Model file for the job. Use its own axes, mm. Coordinates: 2 decimals unless noted, no trailing zeros. Order: outer loops, then holes, each group sorted by start corner. A loop starts at its lowest first (then second) coordinate and runs counter-clockwise, first axis right, second up. Notation, with made-up numbers: (23.25, -39.75) -> (36.25, -39.75) arc R12 ccw to (36.25, -26.75) -> close; hole circle Ø6 at (55.5, 88). An arc over 180 degrees is marked (long way). Use CSV: the item, a comma, the result in double quotes. Start each with the question number.
(1) Cut at C-C on y = 97.5. Write the cut outline in (x, z), plus the area to 3 significant figures.
(2) Cut at B-B on x = 26. Write the cut outline in (y, z), plus the area to 3 significant figures.
(3) Pin check, flat tips, straight feed: pin 1 Ø1.5 at (x, y) = (-29.5, 83) entering from -Z; pin 2 Ø1.5 at (y, z) = (94, 2) entering from +X. Stop position of each tip, or through.
(4) Cut at A-A on z = 1.7. Write the cut outline in (x, y), plus the area to 3 significant figures.
(5) Probe L1, parallel to Y at x = -1, z = 0.4; L2, parallel to Y at x = -0.17, z = 1.5; L3, parallel to Y at x = -48, z = 1.15. List the from-to ranges inside material, lowest first.
(6) Pull direction X, two halves, no side cores. Call faces 1 (the flat face through (-85, 53, 1)), 2 (the flat face through (-1, 66, 3)), 3 (the cylindrical face through (-0.645, 115.504, 1.479)): pulls with the +X half, pulls with the -X half, needs draft (parallel to the pull), parting line crosses it, or undercut.
Autodesk Inventor part; units mm, degrees
ref_plane "YZ Plane" through (0, 0, 0) normal (1, 0, 0) x (0, 1, 0)
ref_plane "XZ Plane" through (0, 0, 0) normal (0, 1, 0) x (-1, 0, 0)
ref_plane "XY Plane" through (0, 0, 0) normal (0, 0, 1) x (1, 0, 0)
sketch "Boceto1" plane through (0, 0, 0) normal (0, 0, 1) x (1, 0, 0)
  arc A0 (-1.5, 113.1763) -> (1.5, 113.1763) centre (0, 113.1763) ccw
  line L0 (0, 113.1763) -> (0, 116.1763)
  line L1 (-75, 45) -> (75, 45)
  line L2 (75, 45) -> (85, 45)
  line L3 (-75, 45) -> (-85, 45)
  line L4 (0, 117.735) -> (-0.0114, 117.7429)
  line L5 (-85, 55) -> (0, 111.6763)
  line L6 (0, 111.6763) -> (85, 55)
  line L7 (-2.22, 113.8018) -> (0.2156, 115.4258)
  line L8 (1.8799, 112.9298) -> (0.2156, 115.4258)
  line L9 (-0.5557, 111.3058) -> (1.8799, 112.9298)
  line L10 (1.8799, 112.9298) -> (0.2156, 115.4258)
  line L11 (-2.22, 113.8018) -> (0.2156, 115.4258)
  line L12 (-0.5557, 111.3058) -> (-2.22, 113.8018)
  line L13 (-2.22, 113.8018) -> (1.8799, 112.9298)
  line L14 (-0.5557, 111.3058) -> (0.2156, 115.4258)
  circle A1 centre (-0.17, 113.3658) radius 2.0958
  line L15 (85, 45) -> (85, 59.843)
  line L16 (-85, 45) -> (-85, 59.843)
  circle A2 centre (-0.17, 113.3658) radius 2.1904
  line L17 (0, 117.0317) -> (-85, 60.3554)
  line L18 (85, 60.3554) -> (0, 117.0317)
  line L19 (-85, 60.3554) -> (-85, 45)
  line L20 (85, 45) -> (85, 60.3554)
  point P0 (0, 0)
  point P1 (96.4858, 46.8907)
  point P2 (-94.6783, 48.1668)
  point P3 (-94.6783, 45)
  point P4 (96.4858, 45)
  dimension "d0" = 3
extrude "Extrusión1" add sketch "Boceto1" along normal blind 3 contours A2 L6 L15 L2 L1 L3 L16 L5 | L5 L16 L19 L17 L18 L20 L15 L6 A2
Outcome:
1,outline,"(-29.29, 0) -> (29.29, 0) -> (29.29, 3) -> (-29.29, 3) -> close"
1,area,"176 mm2"
2,outline,"(45, 0) -> (99.7, 0) -> (99.7, 3) -> (45, 3) -> close"
2,area,"164 mm2"
3,pin 1,"z = 0"
3,pin 2,"x = 35.67"
4,outline,"(-85, 45) -> (85, 45) -> (85, 60.36) -> (0, 117.03) -> (-85, 60.36) -> close; hole circle Ø4.38 at (-0.17, 113.37)"
4,area,"7,410 mm2"
5,L1,"45 to 111.34, 115.39 to 116.36"
5,L2,"45 to 111.18, 115.56 to 116.92"
5,L3,"45 to 85.03"
6,face 1,"pulls with the -X half"
6,face 2,"needs draft"
6,face 3,"undercut"
